Input: part model. Units: mm. Frame: model coordinates. Face numbers are marked on the shaded views. Round coordinates to 2 decimals unless told otherwise and drop trailing zeros. Order: outer loops, then holes, each group sorted by start corner. A loop starts at its lowest first (then second) coordinate and runs counter-clockwise, first axis right, second up. Notation, with made-up numbers: (-29.5, 12.25) - (-20.5, 12.25) arc R34 ccw to (-20.5, 47.25) - close; hole circle Ø9 at (4, 60.25). An arc over 180 degrees is marked (long way). One line per item, written item: value. Start each with the question number.
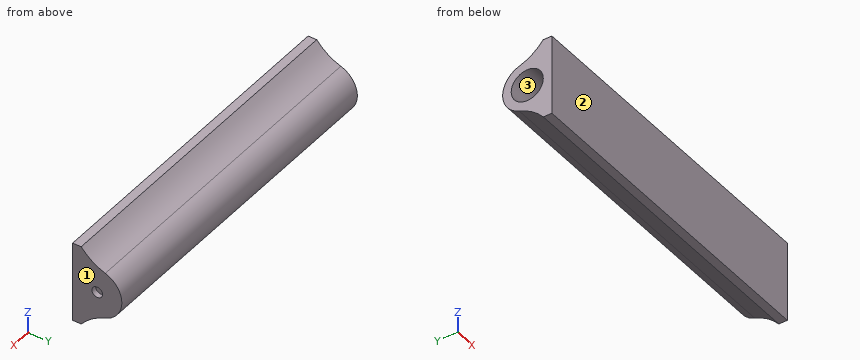
from build123d import *

# Parameters (mm, degrees)
SKETCH2_R           = 3
BOSS_EXTRUDE1_DEPTH = 63
FILLET1_R           = 10
SKETCH4_W           = 1
SKETCH4_H           = 2
LPATTERN1_COUNT     = 27
LPATTERN1_PITCH     = 2


with BuildPart() as part:
    # Sketch2 → Boss-Extrude1 (new body)
    with BuildSketch(Plane(origin=(0, 0, 0), x_dir=(0, 0, -1), z_dir=(1, 0, 0))):
        with BuildLine():
            Line((7.5, 0), (-7.5, 0))
            Line((-7.5, 0), (-7.5, 1.6))
            Line((-7.5, 1.6), (-4.6, 1.6))
            Line((-4.6, 1.6), (-4.6, 4.6))
            ThreePointArc((-4.6, 4.6), (0, 9.2), (4.6, 4.6))
            Line((4.6, 4.6), (4.6, 1.6))
            Line((4.6, 1.6), (7.5, 1.6))
            Line((7.5, 1.6), (7.5, 0))
        make_face()
        with Locations((0, 4.6)):
            Circle(SKETCH2_R, mode=Mode.SUBTRACT)
    extrude(amount=BOSS_EXTRUDE1_DEPTH)

    # Fillet1
    # the kernel refuses this fillet: 10 mm, written as the material it adds along each edge
    with BuildSketch(Plane(origin=(0, 1.6, 4.6), x_dir=(0, 0, 1), z_dir=(1, 0, 0))) as fillet1_piece_1:
        with BuildLine():
            CenterArc((9.2002873, -7.76571825), FILLET1_R, 129.052242215, 31.8961874)
            Line((-0.251964275, -4.501527668), (-1.197189433, -4.17510861))
            ThreePointArc((-1.197189433, -4.17510861), (-1, -3), (-1, 0))
            Line((-1, 0), (0, 1))
            ThreePointArc((0, 1), (1.45, 1), (2.26997127, 0.776571825))
            Line((2.26997127, 0.776571825), (2.9, 0))
        make_face()
    extrude(amount=63)
    with BuildSketch(Plane(origin=(0, 1.6, -4.6), x_dir=(0, 0.9984371795736424, 0.05588558351695166), z_dir=(1, 0, 0))) as fillet1_piece_2:
        with BuildLine():
            CenterArc((7.239418403, -9.619900599), FILLET1_R, 105.847893216, 31.8961874)
            Line((-0.162068192, -2.895467821), (-0.902216852, -2.223024543))
            ThreePointArc((-0.902216852, -2.223024543), (-1.079471276, -1.391848327), (-0.99843718, 0.055885584))
            Line((-0.99843718, 0.055885584), (0.055885584, 0.99843718))
            ThreePointArc((0.055885584, 0.99843718), (3.051197122, 0.830780429), (4.235489295, 0.96199006))
            Line((4.235489295, 0.96199006), (4.508573759, 0))
        make_face()
    extrude(amount=63)

    # Sketch4 → Revolve1 (revolve)
    with BuildSketch(Plane.XY, mode=Mode.PRIVATE) as revolve1_sk:
        with Locations((62.5, 6.6)):
            Rectangle(SKETCH4_W, SKETCH4_H)
    revolve1 = revolve(revolve1_sk.sketch.rotate(Axis((63, 4.6, 0), (-1, 0, 0)), 180), axis=Axis((63, 4.6, 0), (-1, 0, 0)))

    # LPattern1: Revolve1 ×27
    with Locations(*[(-i * LPATTERN1_PITCH, 0, 0) for i in range(1, LPATTERN1_COUNT)]):
        add(revolve1)


solid = part.part
1. Pin query (flat end, axial travel): pin 1 (1.8 mm diameter, centred on y = 4.6, z = 0, fed in from -X); pin 2 (2 mm diameter, centred on y = 2.5, z = -3.5, fed in from -X); pin 3 (5.5 mm diameter, centred on y = 4.6, z = 0, fed in from -X). Return the tip coordinate at first contact, or that it passes through.
2. Section C-C (y = 3). State how many separate pieces and enclosed holes the cut face has, then the cut area to 3 significant figures.
3. Line query: line 1 (Y direction, x = 61.7, z = 0); line 2 (Z direction, x = 27.5, y = 4); line 3 (Y direction, x = 43.5, z = -1.75). Output: solid intervals per line, ascending. Write a range as from..to.
4. Section A-A (z = -5). Return the cut outline in (x, y).
5. Section B-B (y = 8.25). Return the cut outline in (x, z), then the cut area to 3 significant figures.
6. Pull-direction query (Y, two-part tool) for the marked faces 1, 2 and 3; classes: released by +Y, released by -Y, zero draft, split by the parting line, or undercut.
Solved:
1. pin 1: passes through
1. pin 2: stops at x = 0
1. pin 3: stops at x = 10
2. separate pieces: 1
2. enclosed holes: 26
2. area: 584 mm²
3. line 1: y = 0..1.6, 7.6..9.2
3. line 2: z = -5.36..-2.94, 2.94..5.36
3. line 3: y = 0..2.16, 7.04..8.85
4. outline: (0, 0) - (63, 0) - (63, 4.62) - (0, 4.62) - close
5. outline: (0, -2.8) - (63, -2.8) - (63, 2.8) - (0, 2.8) - close
5. area: 353 mm²
6. face 1: zero draft
6. face 2: released by -Y
6. face 3: undercut
